Could you check a few things on this model? Use its own coordinates, in mm. A direction names the side the tool comes from. Coordinates: 2 decimals unless noted, no trailing zeros. Loops run counter-clockwise (first coordinate to the right, second up) from the corner with the lowest first, then second, coordinate; pieces in that order, holes last. Notation, with made-up numbers: (-10.75, 7.5) - (21.25, 7.5) arc R12 ccw to (21.25, 25.5) - close; hole circle Ø3 at (22.25, 75). An arc over 180 degrees is marked (long way). Use CSV: the item, a comma, the result in double quotes.
from build123d import *

# Parameters (mm, degrees)
SZKIC1_W                    = 85.85
SZKIC1_H                    = 85.85
DODANIE_WYCI_GNI_CIE2_DEPTH = 116
SZKIC3_R                    = 36.5
DODANIE_WYCI_GNI_CIE3_DEPTH = 1.6
SZKIC5_W                    = 16.25
SZKIC5_H                    = 16.25
WYTNIJ_WYCI_GNI_CIE1_DEPTH  = 106
SZYK_LINIOWY1_COUNT         = 2
SZYK_LINIOWY1_PITCH         = 69.6
SZYK_LINIOWY1_COUNT_DIR2    = 2
SZYK_LINIOWY1_PITCH_DIR2    = 69.6
SZKIC6_R                    = 2
WYTNIJ_WYCI_GNI_CIE2_DEPTH  = 10
SZYK_LINIOWY2_COUNT         = 2
SZYK_LINIOWY2_PITCH         = 69.6
SZYK_LINIOWY2_COUNT_DIR2    = 2
SZYK_LINIOWY2_PITCH_DIR2    = 69.6
SZKIC7_R                    = 7
DODANIE_WYCI_GNI_CIE4_DEPTH = 35.4
SZKIC8_R                    = 8
SZKIC8_R_2                  = 7
WYTNIJ_WYCI_GNI_CIE5_DEPTH  = 10
ZAOKR_GLENIE1_R             = 5
ZAOKR_GLENIE2_R             = 5
ZAOKR_GLENIE3_R             = 5


with BuildPart() as part:
    # Szkic1 → Dodanie-wyciągnięcie2 (new body)
    with BuildSketch(Plane.XY):
        Rectangle(SZKIC1_W, SZKIC1_H)
    extrude(amount=DODANIE_WYCI_GNI_CIE2_DEPTH)

    # Szkic3 → Dodanie-wyciągnięcie3 (add)
    with BuildSketch(Plane.XY.offset(116)):
        Circle(SZKIC3_R)
    extrude(amount=DODANIE_WYCI_GNI_CIE3_DEPTH)

    # Szkic5 → Wytnij-wyciągnięcie1 (cut)
    with BuildSketch(Plane(origin=(0, 0, 0), x_dir=(-1, 0, 0), z_dir=(0, 0, -1))):
        with Locations((-34.8, 34.8)):
            Rectangle(SZKIC5_W, SZKIC5_H)
    wytnij_wyci_gni_cie1 = extrude(amount=-WYTNIJ_WYCI_GNI_CIE1_DEPTH, mode=Mode.SUBTRACT)

    # Szyk liniowy1: Wytnij-wyci_gni_cie1 2 × 2
    with Locations(*[(-i * SZYK_LINIOWY1_PITCH, -j * SZYK_LINIOWY1_PITCH_DIR2, 0) for i in range(SZYK_LINIOWY1_COUNT) for j in range(SZYK_LINIOWY1_COUNT_DIR2) if (i, j) != (0, 0)]):
        add(wytnij_wyci_gni_cie1, mode=Mode.SUBTRACT)

    # Szkic6 → Wytnij-wyciągnięcie2 (cut)
    with BuildSketch(Plane.XY.offset(116)):
        with Locations((-34.8, 34.8)):
            Circle(SZKIC6_R)
    wytnij_wyci_gni_cie2 = extrude(amount=-WYTNIJ_WYCI_GNI_CIE2_DEPTH, mode=Mode.SUBTRACT)

    # Szyk liniowy2: Wytnij-wyci_gni_cie2 2 × 2
    with Locations(*[(i * SZYK_LINIOWY2_PITCH, -j * SZYK_LINIOWY2_PITCH_DIR2, 0) for i in range(SZYK_LINIOWY2_COUNT) for j in range(SZYK_LINIOWY2_COUNT_DIR2) if (i, j) != (0, 0)]):
        add(wytnij_wyci_gni_cie2, mode=Mode.SUBTRACT)

    # Szkic7 → Dodanie-wyciągnięcie4 (add)
    with BuildSketch(Plane.XY.offset(117.6)):
        Circle(SZKIC7_R)
    extrude(amount=DODANIE_WYCI_GNI_CIE4_DEPTH)

    # Szkic8 → Wytnij-wyciągnięcie5 (cut)
    with BuildSketch(Plane.XY.offset(117.6)):
        Circle(SZKIC8_R)
        Circle(SZKIC8_R_2, mode=Mode.SUBTRACT)
    extrude(amount=-WYTNIJ_WYCI_GNI_CIE5_DEPTH, mode=Mode.SUBTRACT)

    # Zaokrąglenie1
    zaokr_glenie1_edges = [part.edges().sort_by_distance(p)[0] for p in [
        (42.925, -42.925, 111),
        (-42.925, -42.925, 111),
        (-42.925, 42.925, 111),
        (42.925, 42.925, 111),
    ]]
    fillet(zaokr_glenie1_edges, radius=ZAOKR_GLENIE1_R)

    # Zaokrąglenie2
    zaokr_glenie2_edges = [part.edges().sort_by_distance(p)[0] for p in [
        (42.925, 26.675, 53),
        (26.675, 42.925, 53),
        (42.925, -26.675, 53),
        (26.675, -42.925, 53),
        (-26.675, 42.925, 53),
        (-42.925, 26.675, 53),
        (-26.675, -42.925, 53),
        (-42.925, -26.675, 53),
    ]]
    fillet(zaokr_glenie2_edges, radius=ZAOKR_GLENIE2_R)

    # Zaokrąglenie3
    zaokr_glenie3_edges = [part.edges().sort_by_distance(p)[0] for p in [
        (26.675, 26.675, 53),
        (26.675, -26.675, 53),
        (-26.675, 26.675, 53),
        (-26.675, -26.675, 53),
    ]]
    fillet(zaokr_glenie3_edges, radius=ZAOKR_GLENIE3_R)


solid = part.part
(1) Which directions (+Z, -Z, +X, -X, +Y, -Y) give clear straight access to the entire face, cutting with the end or side of a thin tool? Please do faces 1 (the face through (25.17, 41.5, 53.74)), 2 (the face through (-41.5, 25.17, 53.74)), 3 (the face through (-35, -26.675, 52)), 4 (the face through (4, -6, 107.6)).
Computed:
face 1,"-Z, +X, +Y"
face 2,"-Z, -X, +Y"
face 3,"-Z, -X, -Y"
face 4,"+Z"
(2) Thinking about a two-plate mould opening in Y: for faces 5 (the face through (-32.953, -35.566, 111.07)), 6 (the face through (-26.675, -35, 52)), 7 (the face through (41.5, -25.17, 53.74)), which applies, +Y half, -Y half, draft (parallel to the pull), parting line (faces both ways), or undercut?
Computed:
face 5,"undercut"
face 6,"draft"
face 7,"-Y half"
(3) Suppose I cut it at A-A (y = -34.8). Write out the boundary of the cut face in (x, z) (3 decimals).
Computed:
outline,"(-42.925, 106) - (-36.8, 106) - (-36.8, 116) - (-42.925, 116) - close; (-32.8, 106) - (-26.675, 106) - (-26.675, 0) - (26.675, 0) - (26.675, 106) - (32.8, 106) - (32.8, 116) - (11.01, 116) - (11.01, 117.6) - (-11.01, 117.6) - (-11.01, 116) - (-32.8, 116) - close; (36.8, 106) - (42.925, 106) - (42.925, 116) - (36.8, 116) - close"
(4) Suppose I cut it at D-D (x = 0). Write out the boundary of the cut face in (y, z) (3 decimals), plus the area to 3 significant figures.
Computed:
outline,"(-42.925, 0) - (42.925, 0) - (42.925, 116) - (36.5, 116) - (36.5, 117.6) - (8, 117.6) - (8, 107.6) - (7, 107.6) - (7, 153) - (-7, 153) - (-7, 107.6) - (-8, 107.6) - (-8, 117.6) - (-36.5, 117.6) - (-36.5, 116) - (-42.925, 116) - close"
area,"10,600 mm²"
(5) Please list where these lines run through material, in increasing order: line 1 (Y direction, x = 0, z = 109) (3 decimals); line 2 (Y direction, x = 34.8, z = 112) (3 decimals); line 3 (Z direction, x = -38, y = 4.5).
Computed:
line 1,"y = -42.925 to -8, -7 to 7, 8 to 42.925"
line 2,"y = -42.925 to -36.8, -32.8 to 32.8, 36.8 to 42.925"
line 3,"z = 0 to 116"
(6) Will these pins go through, and if not, where does the flat tip stop? pin 1 (2.5 mm diameter, centred on x = 34.8, y = -34.8, fed in from -Z); pin 2 (1.9 mm diameter, centred on x = 34, z = 67.5, fed in from -Y) (3 decimals); pin 3 (1.9 mm diameter, centred on y = -34.5, z = 48.5, fed in from +X) (3 decimals); pin 4 (2 mm diameter, centred on x = 24, y = 31.5, fed in from +Z).
Computed:
pin 1,"passes through"
pin 2,"stops at y = -26.675"
pin 3,"stops at x = 26.675"
pin 4,"stops at z = 116"
(7) Suppose I cut it at C-C (z = 45). Write out the boundary of the cut face in (x, y) (3 decimals), plus the area to 3 significant figures.
Computed:
outline,"(-42.925, -21.675) arc R5 ccw to (-37.925, -26.675) - (-31.675, -26.675) arc R5 cw to (-26.675, -31.675) - (-26.675, -37.925) arc R5 ccw to (-21.675, -42.925) - (21.675, -42.925) arc R5 ccw to (26.675, -37.925) - (26.675, -31.675) arc R5 cw to (31.675, -26.675) - (37.925, -26.675) arc R5 ccw to (42.925, -21.675) - (42.925, 21.675) arc R5 ccw to (37.925, 26.675) - (31.675, 26.675) arc R5 cw to (26.675, 31.675) - (26.675, 37.925) arc R5 ccw to (21.675, 42.925) - (-21.675, 42.925) arc R5 ccw to (-26.675, 37.925) - (-26.675, 31.675) arc R5 cw to (-31.675, 26.675) - (-37.925, 26.675) arc R5 ccw to (-42.925, 21.675) - close"
area,"6,290 mm²"
